```python
from build123d import *

# Parameters (mm, degrees)
PAD004_DEPTH    = 4
FILLET004_R     = 2.4
POCKET006_DEPTH = 3
SKETCH017_R     = 2.45
PAD012_DEPTH    = 4
SKETCH018_R     = 1.05
POCKET009_DEPTH = 5.001
SKETCH019_R     = 2
POCKET010_DEPTH = 3
PAD013_DEPTH    = 1
SKETCH022_W     = 28
SKETCH022_H     = 3
PAD014_DEPTH    = 3
FILLET009_R     = 1


with BuildPart() as part:
    # Sketch009 (on DatumPlane) → Pad004 (new body)
    with BuildSketch(Plane.XY.offset(6.5)):
        with BuildLine():
            Line((1.4, 47.5), (32.4, 47.5))
            ThreePointArc((35.4, 44.5), (34.52132, 46.62132), (32.4, 47.5))
            Line((35.4, 44.5), (35.4, 1.5))
            ThreePointArc((32.4, -1.5), (34.52132, -0.62132), (35.4, 1.5))
            Line((1.4, -1.5), (32.4, -1.5))
            ThreePointArc((-1.6, 1.5), (-0.72132, -0.62132), (1.4, -1.5))
            Line((-1.6, 44.5), (-1.6, 1.5))
            ThreePointArc((1.4, 47.5), (-0.72132, 46.62132), (-1.6, 44.5))
        make_face()
    extrude(amount=PAD004_DEPTH)

    # Fillet004
    fillet004_edges = [part.edges().sort_by_distance(p)[0] for p in [
        (16.9, 47.5, 10.5),
    ]]
    fillet(fillet004_edges, radius=FILLET004_R)

    # Sketch010 (on Face4 of Fillet004) → Pocket006 (cut)
    with BuildSketch(Plane(origin=(0, 0, 6.5), x_dir=(1, 0, 0), z_dir=(0, 0, -1))):
        with BuildLine():
            ThreePointArc((2.4, -0.5), (0.985786, -1.085786), (0.4, -2.5))
            Line((0.4, -2.5), (0.4, -43.5))
            ThreePointArc((0.4, -43.5), (0.985792, -44.914219), (2.400016, -45.5))
            Line((31.4, -45.5), (2.400016, -45.5))
            ThreePointArc((31.4, -45.5), (32.814214, -44.914214), (33.4, -43.5))
            Line((33.4, -2.5), (33.4, -43.5))
            ThreePointArc((33.4, -2.5), (32.814214, -1.085786), (31.4, -0.5))
            Line((2.4, -0.5), (31.4, -0.5))
        make_face()
    extrude(amount=-POCKET006_DEPTH, mode=Mode.SUBTRACT)

    # Sketch017 (on Face27 of Pocket006) → Pad012 (join)
    with BuildSketch(Plane(origin=(0, 0, 9.5), x_dir=(1, 0, 0), z_dir=(0, 0, -1))):
        with Locations((5.9, -3)):
            Circle(SKETCH017_R)
        with Locations((27.9, -3)):
            Circle(SKETCH017_R)
        with Locations((5.9, -42.96)):
            Circle(SKETCH017_R)
        with Locations((27.9, -42.96)):
            Circle(SKETCH017_R)
    extrude(amount=PAD012_DEPTH)

    # Sketch018 (on Face34 of Pad012) → Pocket009 (cut, through all)
    with BuildSketch(Plane(origin=(0, 0, 5.5), x_dir=(1, 0, 0), z_dir=(0, 0, -1))):
        with Locations((5.9, -3)):
            Circle(SKETCH018_R)
        with Locations((27.9, -3)):
            Circle(SKETCH018_R)
        with Locations((5.9, -42.96)):
            Circle(SKETCH018_R)
        with Locations((27.9, -42.96)):
            Circle(SKETCH018_R)
    extrude(amount=-POCKET009_DEPTH, mode=Mode.SUBTRACT)

    # Sketch019 (on Face9 of Pocket009) → Pocket010 (cut)
    with BuildSketch(Plane.XY.offset(10.5)):
        with Locations((27.9, 3)):
            Circle(SKETCH019_R)
        with Locations((5.9, 3)):
            Circle(SKETCH019_R)
        with Locations((27.9, 42.96)):
            Circle(SKETCH019_R)
        with Locations((5.9, 42.96)):
            Circle(SKETCH019_R)
    extrude(amount=-POCKET010_DEPTH, mode=Mode.SUBTRACT)

    # Sketch021 (on Face4 of Pocket010) → Pad013 (join)
    with BuildSketch(Plane(origin=(0, 0, 6.5), x_dir=(1, 0, 0), z_dir=(0, 0, -1))):
        with BuildLine():
            ThreePointArc((2.4, 0.15), (0.526163, -0.626172), (-0.25, -2.500013))
            Line((-0.25, -43.5), (-0.25, -2.500013))
            ThreePointArc((-0.25, -43.5), (0.526167, -45.373833), (2.4, -46.15))
            Line((31.4, -46.15), (2.4, -46.15))
            ThreePointArc((31.4, -46.15), (33.273833, -45.373833), (34.05, -43.5))
            Line((34.05, -2.5), (34.05, -43.5))
            ThreePointArc((34.05, -2.5), (33.273833, -0.626167), (31.4, 0.15))
            Line((2.4, 0.15), (31.4, 0.15))
        make_face()
        with BuildLine():
            ThreePointArc((2.4, -0.5), (0.985786, -1.085786), (0.4, -2.5))
            Line((0.4, -43.5), (0.4, -2.5))
            ThreePointArc((0.4, -43.5), (0.985786, -44.914214), (2.4, -45.5))
            Line((31.4, -45.5), (2.4, -45.5))
            ThreePointArc((31.4, -45.5), (32.814214, -44.914214), (33.4, -43.5))
            Line((33.4, -2.5), (33.4, -43.5))
            ThreePointArc((33.4, -2.5), (32.814214, -1.085787), (31.4, -0.5))
            Line((2.4, -0.5), (31.4, -0.5))
        make_face(mode=Mode.SUBTRACT)
    extrude(amount=PAD013_DEPTH)

    # Sketch022 (on Face60 of Pad013) → Pad014 (join)
    with BuildSketch(Plane(origin=(0, 0, 9.5), x_dir=(1, 0, 0), z_dir=(0, 0, -1))):
        with Locations((16.9, -11.48)):
            Rectangle(SKETCH022_W, SKETCH022_H)
        with Locations((16.9, -34.48)):
            Rectangle(SKETCH022_W, SKETCH022_H)
    extrude(amount=PAD014_DEPTH)

    # Fillet009
    fillet009_edges = [part.edges().sort_by_distance(p)[0] for p in [
        (2.9, 12.98, 8),
        (2.9, 9.98, 8),
        (30.9, 9.98, 8),
        (30.9, 12.98, 8),
        (30.9, 32.98, 8),
        (30.9, 35.98, 8),
        (2.9, 35.98, 8),
        (2.9, 32.98, 8),
    ]]
    fillet(fillet009_edges, radius=FILLET009_R)


solid = part.part
```
For this review, take the finished solid that the model builds, in its own axes (mm). A direction names the side the tool comes from. Coordinates: 2 decimals unless noted, no trailing zeros. Loops run counter-clockwise (first coordinate to the right, second up) from the corner with the lowest first, then second, coordinate; pieces in that order, holes last.
1. Insertion check: P1, Ø2.5, axis at x = 5.9, y = 42.96, coming from the -Z side; P2, Ø2.5, axis at x = 12.5, y = 11, coming from the -Z side; P3, Ø1.5, axis at x = 14.5, z = 9.5, coming from the -Y side; P4, Ø3.5, axis at x = 5.9, y = 3, coming from the +Z side. Each pin has a flat end and moves straight along its axis. Give the tip position at first contact, or say it passes through.
2. Add section C-C, the plane x = 27.9. Count the separate pieces of the cut face and the enclosed holes in it, then the cut area to 3 significant figures.
3. Mouldability with a two-part tool opening along Y and no side actions: class faces 1 (the flat face through (30.9, 34.5, 8)), 2 (the cylindrical face through (-0.7, 46.64, 7.29)), 3 (the flat face through (35.4, 23, 7)) as +Y half, -Y half, draft (parallel to the pull), parting line (faces both ways), or undercut.
4. Add section B-B, the plane y = 14.5. Give the boundary of the cut face in (x, z), then the cut area to 3 significant figures.
5. For faces 4 (the flat face through (2.9, 11.5, 8)), 5 (the flat face through (34.05, 23, 6)), 6 (the flat face through (17, 46.15, 6)), list the 3-axis set-ups (+Z, -Z, +X, -X, +Y, -Y) from which the entire face can be reached by the end or side of a thin tool; tool diameter is ignored.
6. For line 1 (X direction, y = 3, z = 6.6); line 2 (Y direction, x = 21.5, z = 6.8); line 3 (X direction, y = 42.96, z = 6.05), list the stretches that pass through material, from the lowest coordinate up.
7. Add section A-A, the plane x = 21.5. Give the boundary of the cut face in (y, z).
Result:
1. P1: stops at z = 5.5
1. P2: stops at z = 6.5
1. P3: stops at y = -1.41
1. P4: stops at z = 7.5
2. separate pieces: 3
2. enclosed holes: 0
2. area: 84.6 mm2
3. face 1: undercut
3. face 2: +Y half
3. face 3: draft
4. outline: (-1.6, 6.5) - (-0.25, 6.5) - (-0.25, 5.5) - (0.4, 5.5) - (0.4, 9.5) - (33.4, 9.5) - (33.4, 5.5) - (34.05, 5.5) - (34.05, 6.5) - (35.4, 6.5) - (35.4, 8.1) arc R2.4 ccw to (33, 10.5) - (0.8, 10.5) arc R2.4 ccw to (-1.6, 8.1) - close
4. area: 47.8 mm2
5. face 4: -Z
5. face 5: -Z, +X, +Y, -Y
5. face 6: -Z, +X, -X, +Y
6. line 1: x = -1.6 to 0.4, 3.45 to 4.85, 6.95 to 8.35, 25.45 to 26.85, 28.95 to 30.35, 33.4 to 35.4
6. line 2: y = -1.5 to 0.5, 9.98 to 12.98, 32.98 to 35.98, 45.5 to 47.5
6. line 3: x = -0.25 to 0.4, 3.45 to 4.85, 6.95 to 8.35, 25.45 to 26.85, 28.95 to 30.35, 33.4 to 34.05
7. outline: (-1.5, 6.5) - (-0.15, 6.5) - (-0.15, 5.5) - (0.5, 5.5) - (0.5, 9.5) - (9.98, 9.5) - (9.98, 6.5) - (12.98, 6.5) - (12.98, 9.5) - (32.98, 9.5) - (32.98, 6.5) - (35.98, 6.5) - (35.98, 9.5) - (45.5, 9.5) - (45.5, 5.5) - (46.15, 5.5) - (46.15, 6.5) - (47.5, 6.5) - (47.5, 8.1) arc R2.4 ccw to (45.1, 10.5) - (0.9, 10.5) arc R2.4 ccw to (-1.5, 8.1) - close
